Build history of the part. All positions in model axes, mm. A direction names the side the tool comes from. Round coordinates to 2 decimals unless told otherwise and drop trailing zeros. Loops run counter-clockwise (first coordinate to the right, second up) from the corner with the lowest first, then second, coordinate; pieces in that order, holes last. Notation, with made-up numbers: M 44.25,37.5 L 92.25,37.5 A23 cw 92.25,73.5 Z; hole C -37.5,89.25 d3. An arc over 180 degrees is marked long. One line per item, written item: value.
```python
from build123d import *

# Parameters (mm, degrees)
SKETCH_1_R      = 2
SKETCH_1_R_2    = 1.5
SKETCH_1_R_3    = 1
EXTRUDE_1_DEPTH = 3
FILLET_1_R      = 1
FILLET_2_R      = 1


with BuildPart() as part:
    # 草图1 → 凸台-拉伸1 (new body)
    with BuildSketch(Plane.XY):
        with BuildLine():
            Line((0, 7.5), (5, 7.5))
            Line((5, 7.5), (5, 10.5))
            Line((5, 10.5), (15, 10.5))
            Line((15, 10.5), (15, 7.5))
            Line((15, 7.5), (35, 7.5))
            Line((35, 7.5), (35, 10.5))
            Line((35, 10.5), (45, 10.5))
            Line((45, 10.5), (45, 7.5))
            Line((45, 7.5), (54.330127019, 7.5))
            ThreePointArc((54.330127019, 7.5), (55.624222244, 7.670370869), (56.830127019, 8.169872981))
            Line((56.830127019, 8.169872981), (66, 13.464101615))
            ThreePointArc((66, 13.464101615), (70.828427125, 12.828427125), (71.464101615, 8))
            Line((71.464101615, 8), (68.134857418, 2.2335799))
            ThreePointArc((68.134857418, 2.2335799), (67.182681437, 1.047193216), (65.917821708, 0.202040965))
            Line((65.917821708, 0.202040965), (50.405359552, -7.031538935))
            ThreePointArc((50.405359552, -7.031538935), (49.374466313, -7.381480036), (48.292268243, -7.5))
            Line((48.292268243, -7.5), (45, -7.5))
            Line((45, -7.5), (45, -10.5))
            Line((45, -10.5), (35, -10.5))
            Line((35, -10.5), (35, -7.5))
            Line((35, -7.5), (15, -7.5))
            Line((15, -7.5), (15, -10.5))
            Line((15, -10.5), (5, -10.5))
            Line((5, -10.5), (5, -7.5))
            Line((5, -7.5), (0, -7.5))
            Line((0, -7.5), (0, 7.5))
        make_face()
        with Locations((68, 10)):
            Circle(SKETCH_1_R, mode=Mode.SUBTRACT)
        with Locations((5, 0)):
            Circle(SKETCH_1_R_2, mode=Mode.SUBTRACT)
        with Locations((45, 0)):
            Circle(SKETCH_1_R_2, mode=Mode.SUBTRACT)
        with Locations((18, 0)):
            Circle(SKETCH_1_R, mode=Mode.SUBTRACT)
        with Locations((62, 9)):
            Circle(SKETCH_1_R_3, mode=Mode.SUBTRACT)
    extrude(amount=EXTRUDE_1_DEPTH)

    # 圆角1
    fillet_1_edges = [part.edges().sort_by_distance(p)[0] for p in [
        (0, 7.5, 1.5),
        (5, 10.5, 1.5),
        (15, 10.5, 1.5),
        (35, 10.5, 1.5),
        (45, 10.5, 1.5),
        (45, -10.5, 1.5),
        (35, -10.5, 1.5),
        (15, -10.5, 1.5),
        (5, -10.5, 1.5),
        (0, -7.5, 1.5),
    ]]
    fillet(fillet_1_edges, radius=FILLET_1_R)

    # 圆角2
    fillet_2_edges = [part.edges().sort_by_distance(p)[0] for p in [
        (45, -7.5, 1.5),
    ]]
    fillet(fillet_2_edges, radius=FILLET_2_R)


solid = part.part
```
Item 1: Wall check: line 1 along Y through (x, z) = (18, 0.8); line 2 along X through (y, z) = (0.5, 1.05); line 3 along Y through (x, z) = (68, 0.8). Give the ranges that are in metal, low to high.
Check values:
line 1: y = -7.5 to -2, 2 to 7.5
line 2: x = 0 to 3.59, 6.41 to 16.06, 19.94 to 43.59, 46.41 to 66.46
line 3: y = 2.01 to 8, 12 to 14
Item 2: Slice it at B-B, the plane z = 0.45. Give the number of separate pieces and of enclosed holes in the cut face, and give its area (3 significant figures).
Check values:
separate pieces: 1
enclosed holes: 5
area: 1,090 mm2
Item 3: Pull direction Y, two halves, no side cores. Call faces 1 (the face through (43.5, 0.07, 1.48)), 2 (the face through (5, -9, 1)), 3 (the face through (66.526, 11.352, 1.479)), 4 (the face through (69.823, 5.157, 1.479)): pulls with the +Y half, pulls with the -Y half, needs draft (parallel to the pull), parting line crosses it, or undercut.
Check values:
face 1: undercut
face 2: needs draft
face 3: undercut
face 4: pulls with the -Y half
Item 4: Slice it at C-C, the plane y = -5.25. Give the cut face in (x, z).
Check values:
outline: M 0,0 L 54.23,0 L 54.23,3 L 0,3 Z
Item 5: Drop flat-ended pins along their axis: P1, Ø0.6, axis at y = -8, z = 1, coming from the +X side; P2, Ø1, axis at y = -9, z = 2, coming from the -X side; P3, Ø1.5, axis at x = 3, z = 1, coming from the +Y side. Give the stop position or say it passes through.
Check values:
P1: stops at x = 45.4
P2: stops at x = 5
P3: stops at y = 7.5
Item 6: Which spindle directions (+Z, -Z, +X, -X, +Y, -Y) get a long thin tool onto all of the face, cutting with end or side? Do faces 5 (the face through (25, -7.5, 1)), 6 (the face through (3, -7.5, 1)), 7 (the face through (15, 9, 1)). Say none if no direction does.
Check values:
face 5: +Z, -Z, -Y
face 6: +Z, -Z, -X, -Y
face 7: +Z, -Z, +Y
Item 7: Slice it at A-A, the plane x = 33. Give the cut face in (y, z), and give its area (3 significant figures).
Check values:
outline: M -7.5,0 L 7.5,0 L 7.5,3 L -7.5,3 Z
area: 45.0 mm2
